from build123d import *

# Parameters (mm, degrees)
SKETCH1_W           = 25.4
SKETCH1_H           = 25.4
BOSS_EXTRUDE1_DEPTH = 381
SHELL1_T            = -1.5875
SKETCH2_R           = 2.4892
CUT_EXTRUDE1_DEPTH  = 383.689587002
SKETCH3_R           = 2.4892
CUT_EXTRUDE2_DEPTH  = 383.689587002


with BuildPart() as part:
    # Sketch1 → Boss-Extrude1 (new body)
    with BuildSketch(Plane.XY):
        with Locations((12.7, 12.7)):
            Rectangle(SKETCH1_W, SKETCH1_H)
    extrude(amount=-BOSS_EXTRUDE1_DEPTH)

    # Shell1
    shell1_openings = [part.faces().sort_by_distance(p)[0] for p in [
        (12.7, 12.7, -381),
        (12.7, 12.7, 0),
    ]]
    offset(amount=SHELL1_T, openings=shell1_openings, kind=Kind.INTERSECTION)

    # Sketch2 → Cut-Extrude1 (cut, through all)
    with BuildSketch(Plane(origin=(25.4, 0, 0), x_dir=(0, 0, -1), z_dir=(1, 0, 0))):
        with Locations(Location((12.7, 12.7, 0), (0, 0, 90))):
            Circle(SKETCH2_R)
        with Locations(Location((38.1, 12.7, 0), (0, 0, 90))):
            Circle(SKETCH2_R)
        with Locations(Location((63.5, 12.7, 0), (0, 0, 90))):
            Circle(SKETCH2_R)
        with Locations(Location((88.9, 12.7, 0), (0, 0, 90))):
            Circle(SKETCH2_R)
        with Locations(Location((114.3, 12.7, 0), (0, 0, 90))):
            Circle(SKETCH2_R)
        with Locations(Location((139.7, 12.7, 0), (0, 0, 90))):
            Circle(SKETCH2_R)
        with Locations(Location((165.1, 12.7, 0), (0, 0, 90))):
            Circle(SKETCH2_R)
        with Locations(Location((190.5, 12.7, 0), (0, 0, 90))):
            Circle(SKETCH2_R)
        with Locations(Location((215.9, 12.7, 0), (0, 0, 90))):
            Circle(SKETCH2_R)
        with Locations(Location((241.3, 12.7, 0), (0, 0, 90))):
            Circle(SKETCH2_R)
        with Locations(Location((266.7, 12.7, 0), (0, 0, 90))):
            Circle(SKETCH2_R)
        with Locations(Location((292.1, 12.7, 0), (0, 0, 90))):
            Circle(SKETCH2_R)
        with Locations(Location((317.5, 12.7, 0), (0, 0, 90))):
            Circle(SKETCH2_R)
        with Locations(Location((342.9, 12.7, 0), (0, 0, 90))):
            Circle(SKETCH2_R)
        with Locations(Location((368.3, 12.7, 0), (0, 0, 90))):
            Circle(SKETCH2_R)
    extrude(amount=-CUT_EXTRUDE1_DEPTH, mode=Mode.SUBTRACT)

    # Sketch3 → Cut-Extrude2 (cut, through all)
    with BuildSketch(Plane(origin=(0, 25.4, 0), x_dir=(1, 0, 0), z_dir=(0, 1, 0))):
        with Locations(Location((12.7, 12.7, 0), (0, 0, 270))):
            Circle(SKETCH3_R)
        with Locations(Location((12.7, 38.1, 0), (0, 0, 270))):
            Circle(SKETCH3_R)
        with Locations(Location((12.7, 63.5, 0), (0, 0, 270))):
            Circle(SKETCH3_R)
        with Locations(Location((12.7, 88.9, 0), (0, 0, 270))):
            Circle(SKETCH3_R)
        with Locations(Location((12.7, 114.3, 0), (0, 0, 270))):
            Circle(SKETCH3_R)
        with Locations(Location((12.7, 139.7, 0), (0, 0, 270))):
            Circle(SKETCH3_R)
        with Locations(Location((12.7, 165.1, 0), (0, 0, 270))):
            Circle(SKETCH3_R)
        with Locations(Location((12.7, 190.5, 0), (0, 0, 270))):
            Circle(SKETCH3_R)
        with Locations(Location((12.7, 215.9, 0), (0, 0, 270))):
            Circle(SKETCH3_R)
        with Locations(Location((12.7, 241.3, 0), (0, 0, 270))):
            Circle(SKETCH3_R)
        with Locations(Location((12.7, 266.7, 0), (0, 0, 270))):
            Circle(SKETCH3_R)
        with Locations(Location((12.7, 292.1, 0), (0, 0, 270))):
            Circle(SKETCH3_R)
        with Locations(Location((12.7, 317.5, 0), (0, 0, 270))):
            Circle(SKETCH3_R)
        with Locations(Location((12.7, 342.9, 0), (0, 0, 270))):
            Circle(SKETCH3_R)
        with Locations(Location((12.7, 368.3, 0), (0, 0, 270))):
            Circle(SKETCH3_R)
    extrude(amount=-CUT_EXTRUDE2_DEPTH, mode=Mode.SUBTRACT)


solid = part.part
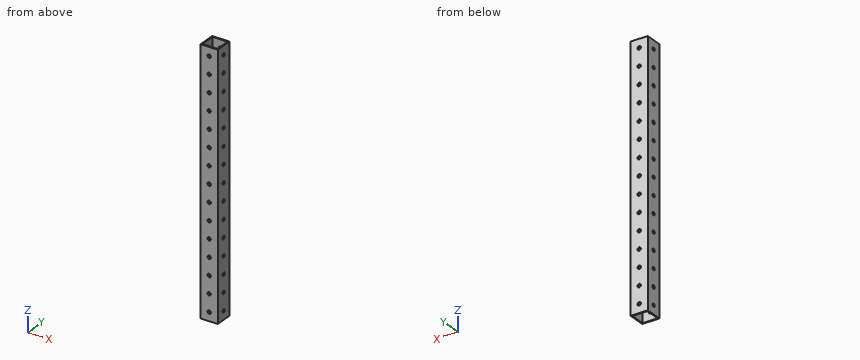
Input: part model. Units: mm. Frame: model coordinates. Coordinates: 2 decimals unless noted, no trailing zeros. Order: outer loops, then holes, each group sorted by start corner. A loop starts at its lowest first (then second) coordinate and runs counter-clockwise, first axis right, second up. Notation, with made-up numbers: M 78,18.5 L 86,18.5 A19 cw 86,24.5 Z; hole C -12.5,82 d9. An arc over 180 degrees is marked long. One line per question, with ' | ' between items.
Item 1: Pin query (flat end, axial travel): pin 1 (3 mm diameter, centred on x = 12.7, z = -12.7, fed in from -Y). Return the tip coordinate at first contact, or that it passes through.
Geometry results:
pin 1: passes through
Item 2: Ray query, line 1 along Y through (x, z) = (7.25, -133); line 2 along X through (y, z) = (1.25, -114.3). Return the intervals inside material, ascending.
Geometry results:
line 1: y = 0 to 1.59, 23.81 to 25.4 | line 2: x = 0 to 10.21, 15.19 to 25.4
Item 3: Section A-A (z = -130.5). Output: boundary loops of the cut face in (x, y), then the cut area to 3 significant figures.
Geometry results:
outline: M 0,0 L 25.4,0 L 25.4,25.4 L 0,25.4 Z; hole M 1.59,1.59 L 23.81,1.59 L 23.81,23.81 L 1.59,23.81 Z | area: 151 mm^2
Item 4: Section B-B (y = 20.5). Output: boundary loops of the cut face in (x, z).
Geometry results:
outline: M 0,-381 L 1.59,-381 L 1.59,0 L 0,0 Z; M 23.81,-381 L 25.4,-381 L 25.4,0 L 23.81,0 Z
